from build123d import *

# Parameters (mm, degrees)
F0_W     = 1000
F0_H     = 300
F1_DEPTH = 1200
F2_W     = 400
F2_H     = 80
F3_DEPTH = 120
F4_W     = 900
F4_H     = 400
F5_DEPTH = 300


with BuildPart() as f1:
    # F0 (on Top) → F1 (new body)
    with BuildSketch(Plane.XY):
        with Locations((-2.975285, 0)):
            Rectangle(F0_W, F0_H)
    extrude(amount=F1_DEPTH)

    # F2 (on face) → F3 (cut)
    with BuildSketch(Plane.XZ.offset(150)):
        with Locations((-252.975285, 640)):
            Rectangle(F2_W, F2_H)
        with Locations((-252.975285, 540)):
            Rectangle(F2_W, F2_H)
        with Locations((-252.975285, 440)):
            Rectangle(F2_W, F2_H)
        with Locations((-252.975285, 340)):
            Rectangle(F2_W, F2_H)
        with Locations((-252.975285, 240)):
            Rectangle(F2_W, F2_H)
    extrude(amount=-F3_DEPTH, mode=Mode.SUBTRACT)

    # F4 (on face) → F5 (cut)
    with BuildSketch(Plane.XZ.offset(150)):
        with Locations((-2.975285, 941.9734)):
            Rectangle(F4_W, F4_H)
    extrude(amount=-F5_DEPTH, mode=Mode.SUBTRACT)


solid = f1.part
The listing builds one solid part. Answer for the finished solid, in the listing's coordinates (mm). A direction names the side the tool comes from. Coordinates: 2 decimals unless noted, no trailing zeros. Loops run counter-clockwise (first coordinate to the right, second up) from the corner with the lowest first, then second, coordinate; pieces in that order, holes last. Notation, with made-up numbers: M 26,5 L 45,5 A21 ccw 45,36 Z; hole C -33,6 d9. An arc over 180 degrees is marked long. Answer in a Markdown table with one row per item.
1) Given pin 1 (24 mm diameter, centred on x = -337, z = 536.5, fed in from -Y), flat-ended and moving along its own axis, determine where the tip first touches the part or whether it passes through.
Answers below:
| item | result |
|---|---|
| pin 1 | y = -30 |
2) Find section A-A (x = 287). Determine the outline of the cut face in (y, z), then the cut area to 3 significant figures.
Answers below:
| item | result |
|---|---|
| outline | M -150,0 L 150,0 L 150,741.97 L -150,741.97 Z; M -150,1141.97 L 150,1141.97 L 150,1200 L -150,1200 Z |
| area | 240,000 mm^2 |
3) Which of the six approach directions +Z, -Z, +X, -X, +Y, -Y give full straight-line access (tool end or side, diameter ignored) to faces 4 (the flat face through (-502.975, -2, 592)), 5 (the flat face through (-9, -2, 741.973)), 6 (the flat face through (-256, -30, 341))?
Answers below:
| item | result |
|---|---|
| face 4 | +Z, -Z, -X, +Y, -Y |
| face 5 | +Y, -Y |
| face 6 | -Y |
4) Find section B-B (z = 782). Determine the outline of the cut face in (x, y).
Answers below:
| item | result |
|---|---|
| outline | M -502.98,-150 L -452.98,-150 L -452.98,150 L -502.98,150 Z; M 447.02,-150 L 497.02,-150 L 497.02,150 L 447.02,150 Z |
5) Determine the mould class of faces 1 (the flat face through (497.025, -2, 592)), 2 (the flat face through (-10, -150, 458)), 3 (the flat face through (-256, -30, 541)) for opening direction X: released by +X, released by -X, zero draft, split by the parting line, or undercut.
Answers below:
| item | result |
|---|---|
| face 1 | released by +X |
| face 2 | zero draft |
| face 3 | undercut |
6) Find section C-C (y = 79). Determine the outline of the cut face in (x, z), then the cut area to 3 significant figures.
Answers below:
| item | result |
|---|---|
| outline | M -502.98,0 L 497.02,0 L 497.02,1200 L -502.98,1200 Z; hole M -452.98,741.97 L 447.02,741.97 L 447.02,1141.97 L -452.98,1141.97 Z |
| area | 840,000 mm^2 |
7) Find the intervals of material crossed by probe 1 along Z at (x, y) = (9, -14); probe 2 along X at (y, z) = (31, 860); probe 3 along X at (y, z) = (-122.5, 321), in increasing order.
Answers below:
| item | result |
|---|---|
| probe 1 | 0 to 741.97, 1141.97 to 1200 |
| probe 2 | -502.98 to -452.98, 447.02 to 497.02 |
| probe 3 | -502.98 to -452.98, -52.98 to 497.02 |
8) Find section D-D (z = 424.5). Determine the outline of the cut face in (x, y), then the cut area to 3 significant figures.
Answers below:
| item | result |
|---|---|
| outline | M -502.98,-150 L -452.98,-150 L -452.98,-30 L -52.98,-30 L -52.98,-150 L 497.02,-150 L 497.02,150 L -502.98,150 Z |
| area | 252,000 mm^2 |
